Read the model definition and answer for the solid it produces. Units are mm, in the model's axes. A direction names the side the tool comes from. Coordinates: 2 decimals unless noted, no trailing zeros. Order: outer loops, then holes, each group sorted by start corner. A loop starts at its lowest first (then second) coordinate and runs counter-clockwise, first axis right, second up. Notation, with made-up numbers: (1, -31) -> (13, -31) arc R16 ccw to (13, -17) -> close; hole circle Ø2 at (67.25, -28.75). An arc over 180 degrees is marked (long way). Use CSV: the item, a comma, the result in double quotes.
```python
from build123d import *

# Parameters (mm, degrees)
F0_W     = 14.5
F0_H     = 3
F1_DEPTH = 2.5
F2_DEPTH = 9
F3_R     = 1.5606676117
F4_DEPTH = 25
F5_SIZE  = 2.7
F6_R     = 6.5


with BuildPart() as f1:
    # F0 (on Top) → F1 (new body)
    with BuildSketch(Plane.XY):
        Polygon((-15.1000638381, 3.0731637962), (-14.5, 10.1), (-14.5, 14.7897112858), (-16.3062401116, 22.7), (-14.5, 30.5), (-14.5, 33), (-16.8, 43.1), (-18, 43.1), (-18, 40.6315773726), (-15.569419682, 31.8290367723), (-18, 22.7700328082), (-18, 19.7484236718), (-16.0118928999, 12.6614226028), (-18, 3.0642349739), align=None)
        with Locations((-7.25, 1.5)):
            Rectangle(F0_W, F0_H)
        Polygon((-18, 0), (-14.5, 0), (-14.5, 3), (-15.1000638381, 3.0731637962), (-18, 3.0642349739), align=None)
        with Locations((7.25, 1.5)):
            Rectangle(F0_W, F0_H)
        Polygon((14.5, 3), (14.5, 0), (18, 0), (18, 3.0642349739), (15.1000638381, 3.0731637962), align=None)
        Polygon((14.5, 14.7897112858), (14.5, 10.1), (15.1000638381, 3.0731637962), (18, 3.0642349739), (16.0118928999, 12.6614226028), (18, 19.7484236718), (18, 22.7700328082), (15.569419682, 31.8290367723), (18, 40.6315773726), (18, 43.1), (16.8, 43.1), (14.5, 33), (14.5, 30.5), (16.3062401116, 22.7), align=None)
        with BuildLine():
            Line((13.6, 10.1), (14.5, 10.1))
            Line((14.5, 10.1), (14.5, 14.7897112858))
            Line((14.5, 14.7897112858), (14, 12.6))
            add(Edge.make_bspline(
                [(13.6, 10.1), (13.6104541942, 11.4760398865), (13.5792037472, 12.4339209869), (14, 12.6)],
                knots=[0, 0, 0, 0, 2.5317977802, 2.5317977802, 2.5317977802, 2.5317977802], degree=3))
        make_face()
        with BuildLine():
            Line((-14.5, 14.7897112858), (-14.5, 10.1))
            Line((-14.5, 10.1), (-13.6, 10.1))
            add(Edge.make_bspline(
                [(-13.6, 10.1), (-13.6104541942, 11.4760398865), (-13.5792037472, 12.4339209869), (-14, 12.6)],
                knots=[0, 0, 0, 0, 2.5317977802, 2.5317977802, 2.5317977802, 2.5317977802], degree=3))
            Line((-14, 12.6), (-14.5, 14.7897112858))
        make_face()
        with BuildLine():
            Line((18, 22.7700328082), (18, 19.7484236718))
            Line((18, 19.7484236718), (18.3, 20.8178330213))
            Line((18.3, 20.8178330213), (19.2, 20.8178330213))
            add(Edge.make_bspline(
                [(18, 22.7700328082), (18.5130968392, 22.7131574929), (19.1960260391, 22.1627136484), (19.2, 20.8178330213)],
                knots=[0, 0, 0, 0, 2.2915243852, 2.2915243852, 2.2915243852, 2.2915243852], degree=3))
        make_face()
        with BuildLine():
            Line((-18.3, 20.8178330213), (-18, 19.7484236718))
            Line((-18, 19.7484236718), (-18, 22.7700328082))
            add(Edge.make_bspline(
                [(-18, 22.7700328082), (-18.5130968392, 22.7131574929), (-19.1960260391, 22.1627136484), (-19.2, 20.8178330213)],
                knots=[0, 0, 0, 0, 2.2915243852, 2.2915243852, 2.2915243852, 2.2915243852], degree=3))
            Line((-19.2, 20.8178330213), (-18.3, 20.8178330213))
        make_face()
        with BuildLine():
            Line((12.9, 30.5), (14.5, 30.5))
            Line((14.5, 30.5), (14.5, 33))
            add(Edge.make_bspline(
                [(14.5, 33), (13.9373009205, 32.9109020531), (12.9039739609, 31.8448806271), (12.9, 30.5)],
                knots=[0, 0, 0, 0, 2.9681644159, 2.9681644159, 2.9681644159, 2.9681644159], degree=3))
        make_face()
        with BuildLine():
            Line((-14.5, 33), (-14.5, 30.5))
            Line((-14.5, 30.5), (-12.9, 30.5))
            add(Edge.make_bspline(
                [(-14.5, 33), (-13.9373009205, 32.9109020531), (-12.9039739609, 31.8448806271), (-12.9, 30.5)],
                knots=[0, 0, 0, 0, 2.9681644159, 2.9681644159, 2.9681644159, 2.9681644159], degree=3))
        make_face()
        with BuildLine():
            Line((-19.7963143, 40.7467074541), (-18, 40.6315773726))
            Line((-18, 40.6315773726), (-18, 43.1))
            add(Edge.make_bspline(
                [(-18, 43.1), (-18.5130959079, 43.0794730783), (-19.7923403391, 42.0915880812), (-19.7963143, 40.7467074541)],
                knots=[0, 0, 0, 0, 2.9605288161, 2.9605288161, 2.9605288161, 2.9605288161], degree=3))
        make_face()
        with BuildLine():
            Line((18, 43.1), (18, 40.6315773726))
            Line((18, 40.6315773726), (19.7963143, 40.7467074541))
            add(Edge.make_bspline(
                [(18, 43.1), (18.5130959079, 43.0794730783), (19.7923403391, 42.0915880812), (19.7963143, 40.7467074541)],
                knots=[0, 0, 0, 0, 2.9605288161, 2.9605288161, 2.9605288161, 2.9605288161], degree=3))
        make_face()
    extrude(amount=F1_DEPTH)

    # F0 (on Top) → F2 (join)
    with BuildSketch(Plane.XY):
        Polygon((-18, 0), (-14.5, 0), (-14.5, 3), (-15.1000638381, 3.0731637962), (-18, 3.0642349739), align=None)
        with Locations((-7.25, 1.5)):
            Rectangle(F0_W, F0_H)
        with Locations((7.25, 1.5)):
            Rectangle(F0_W, F0_H)
        Polygon((14.5, 3), (14.5, 0), (18, 0), (18, 3.0642349739), (15.1000638381, 3.0731637962), align=None)
    extrude(amount=F2_DEPTH)

    # F3 (on Front) → F4 (cut)
    with BuildSketch(Plane.XZ):
        with Locations((7.4880118482, 4.3315729126)):
            Circle(F3_R)
        with Locations((-7.4880118482, 4.3315729126)):
            Circle(F3_R)
    extrude(amount=-F4_DEPTH, mode=Mode.SUBTRACT)

    # F5
    f5_edges = [f1.edges().sort_by_distance(p)[0] for p in [
        (5.927344, 3, 4.331573),
        (-9.048679, 3, 4.331573),
    ]]
    chamfer(f5_edges, length=F5_SIZE)

    # F6
    f6_edges = [f1.edges().sort_by_distance(p)[0] for p in [
        (-18, 1.532117, 9),
        (18, 1.532117, 9),
    ]]
    fillet(f6_edges, radius=F6_R)


solid = f1.part
```
Item 1: Find section B-B, the plane z = 5. Give the number of separate pieces and of enclosed holes in the cut face, then the cut area to 3 significant figures.
Return value:
separate pieces,"3"
enclosed holes,"0"
area,"73.2 mm^2"
Item 2: Each of these flat-tipped pins is pushed along its axis until it touches: P1, Ø2, axis at y = 35.5, z = 2, coming from the +X side; P2, Ø4, axis at x = 7.49, z = 4.33, coming from the -Y side; P3, Ø2, axis at y = 29.5, z = 2.5, coming from the +X side; P4, Ø1.9, axis at x = -7.49, z = 4.33, coming from the +Y side. Where does it stop, or does it pass through?
Return value:
P1,"stops at x = 16.86"
P2,"stops at y = 0"
P3,"stops at x = 16.46"
P4,"passes through"
Item 3: Find section D-D, the plane y = 27.5. Give the vertices of the cut face in (x, z).
Return value:
outline,"(-16.73, 0) -> (-15.19, 0) -> (-15.19, 2.5) -> (-16.73, 2.5) -> close; (15.19, 0) -> (16.73, 0) -> (16.73, 2.5) -> (15.19, 2.5) -> close"
Item 4: Straight lines are drawn through the part: line 1 along Y through (x, z) = (3, 5.75); line 2 along X through (y, z) = (13, 1.75); line 3 along X through (y, z) = (39.5, 0.5). For each, find the intervals that lie inside material, in ascending order.
Return value:
line 1,"y = 0 to 3"
line 2,"x = -16.11 to -14.09, 14.09 to 16.11"
line 3,"x = -17.69 to -15.98, 15.98 to 17.69"
Item 5: Find section C-C, the plane x = 0. Give the vertices of the cut face in (y, z).
Return value:
outline,"(0, 0) -> (3, 0) -> (3, 9) -> (0, 9) -> close"
Item 6: Find section A-A, the plane y = 9.5. Give the vertices of the cut face in (x, z), then the cut area to 3 significant figures.
Return value:
outline,"(-16.67, 0) -> (-14.55, 0) -> (-14.55, 2.5) -> (-16.67, 2.5) -> close; (14.55, 0) -> (16.67, 0) -> (16.67, 2.5) -> (14.55, 2.5) -> close"
area,"10.6 mm^2"
Item 7: The mould has two halves that part along Y. Classify faces 1 (the flat face through (18, 2, 1)), 2 (the flat face through (-14, 10.1, 1)), 3 (the flat face through (-17, 43.1, 1)), 4 (the flat face through (14, 30.5, 1)): +Y half, -Y half, draft (parallel to the pull), parting line (faces both ways), or undercut.
Return value:
face 1,"draft"
face 2,"undercut"
face 3,"+Y half"
face 4,"undercut"
Item 8: A tool of negligible diameter and unlimited length cuts with its end or side. For faces 5 (the flat face through (-18, 2, 1)), 6 (the flat face through (14, 10.1, 1)), 7 (the flat face through (18.89, 40.69, 1.23)), 8 (the flat face through (15.666, 38.121, 1.232)), 9 (the flat face through (-16.77, 27.36, 1.23)), from which of +Z, -Z, +X, -X, +Y, -Y can it reach the whole face along a straight path? Write none if from no direction.
Return value:
face 5,"+Z, -Z, -X, -Y"
face 6,"+Z, -Z"
face 7,"+Z, -Z, +X"
face 8,"+Z, -Z, +Y"
face 9,"+Z, -Z, -X"
